Could you check a few things on this model? Use its own coordinates, in mm. Face numbers are marked on the shaded views. Round coordinates to 2 decimals unless told otherwise and drop trailing zeros. Write each loop counter-clockwise with the first axis right and the second up, starting at its lowest first coordinate (ties: lowest second). Pieces come first, ordered by that corner, then holes. Notation, with made-up numbers: (19.25, 57.5) - (75.25, 57.5) arc R31 ccw to (75.25, 84.5) - close; hole circle Ø4 at (62.5, 75). An arc over 180 degrees is marked (long way). Write each question's results on one line, items separated by ' | '. Start each with the question number.
(1) Imagine slicing it at D-D on z = 1. Write out the boundary of the cut face in (x, y) (3 decimals), then the cut area to 3 significant figures.
(2) Imagine slicing it at C-C on y = -6. Write out the boundary of the cut face in (x, z), then the cut area to 3 significant figures.
(3) Imagine slicing it at B-B on x = 25.4. Write out the boundary of the cut face in (y, z) (1 decimal), then the cut area to 3 significant figures.
(4) For P1, Ø8, axis at x = 25.4, y = -9.525, coming from the +Z side; P2, Ø4, axis at x = -6, y = -9.5, coming from the +Z side, each with a flat end and sliding along its axis, tell me the tip position at first contact or that it passes through.
(5) Imagine slicing it at A-A on x = -25.4. Write out the boundary of the cut face in (y, z) (1 decimal), then the cut area to 3 significant figures.
(6) Thinking about a two-plate mould opening in X: for the marked faces 1 and 2, which applies, +X half, -X half, draft (parallel to the pull), parting line (faces both ways), or undercut?
(7) Please list where these lines run through material, in increasing order: line 1 (Y direction, x = -25.4, z = 1.6) (3 decimals); line 2 (Y direction, x = 2, z = 1.45) (3 decimals); line 3 (X direction, y = 8.5, z = 1.8). Write a range as [from, to].
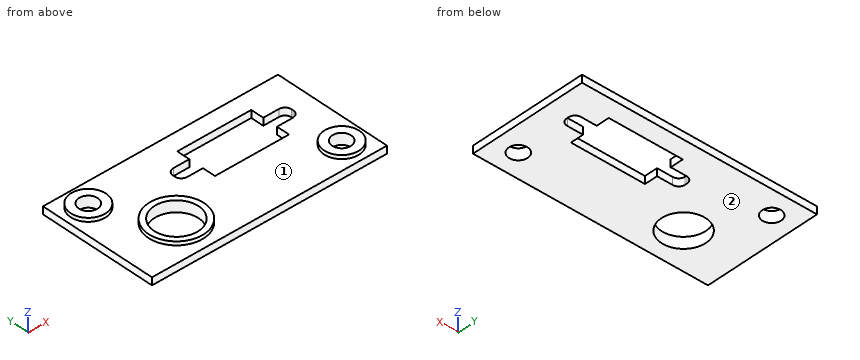
```python
from build123d import *

# Parameters (mm, degrees)
F0_W      = 63.5
F0_H      = 31.75
F1_DEPTH  = 2
F3_R      = 4.7625
F4_DEPTH  = 1
F6_R      = 2.54
F7_DEPTH  = 25.4
F8_W      = 20
F8_H      = 11
F9_DEPTH  = 25
F11_R     = 7.5
F12_DEPTH = 1
F13_R     = 6
F14_DEPTH = 25
F5_R      = 4.7625
F15_DEPTH = 1
F16_R     = 2.54
F17_DEPTH = 25.4
F19_DEPTH = 25


with BuildPart() as f1:
    # F0 (on Top) → F1 (new body)
    with BuildSketch(Plane.XY):
        Rectangle(F0_W, F0_H)
    extrude(amount=F1_DEPTH)

    # F3 (on face) → F4 (join)
    with BuildSketch(Plane.XY.offset(2)):
        with Locations((-25.4, 9.525)):
            Circle(F3_R)
    extrude(amount=F4_DEPTH)

    # F6 (on face) → F7 (cut)
    with BuildSketch(Plane.XY.offset(3)):
        with Locations((-25.4, 9.525)):
            Circle(F6_R)
    extrude(amount=-F7_DEPTH, mode=Mode.SUBTRACT)

    # F8 (on face) → F9 (cut)
    with BuildSketch(Plane.XY.offset(2)):
        with Locations((10, 5.5)):
            Rectangle(F8_W, F8_H)
    extrude(amount=-F9_DEPTH, mode=Mode.SUBTRACT)

    # F11 (on face) → F12 (join)
    with BuildSketch(Plane.XY.offset(2)):
        with Locations((-16, -6)):
            Circle(F11_R)
    extrude(amount=F12_DEPTH)

    # F13 (on face) → F14 (cut)
    with BuildSketch(Plane.XY.offset(3)):
        with Locations((-16, -6)):
            Circle(F13_R)
    extrude(amount=-F14_DEPTH, mode=Mode.SUBTRACT)

    # F5 (on face) → F15 (join)
    with BuildSketch(Plane.XY.offset(2)):
        with Locations((25.4, -9.525)):
            Circle(F5_R)
    extrude(amount=F15_DEPTH)

    # F16 (on face) → F17 (cut)
    with BuildSketch(Plane.XY.offset(3)):
        with Locations((25.4, -9.525)):
            Circle(F16_R)
    extrude(amount=-F17_DEPTH, mode=Mode.SUBTRACT)

    # F18 (on face) → F19 (cut)
    with BuildSketch(Plane.XY.offset(2)):
        with BuildLine():
            Line((6, 3.5), (6, 7.5))
            Line((6, 7.5), (-4.25, 7.5))
            ThreePointArc((-4.25, 7.5), (-5.487437, 6.987437), (-6, 5.75))
            Line((-6, 5.75), (-6, 5.25))
            ThreePointArc((-6, 5.25), (-5.487437, 4.012563), (-4.25, 3.5))
            Line((-4.25, 3.5), (6, 3.5))
        make_face()
        with BuildLine():
            Line((14, 3.5), (24.25, 3.5))
            ThreePointArc((24.25, 3.5), (25.487437, 4.012563), (26, 5.25))
            Line((26, 5.25), (26, 5.75))
            ThreePointArc((26, 5.75), (25.487437, 6.987437), (24.25, 7.5))
            Line((24.25, 7.5), (14, 7.5))
            Line((14, 7.5), (14, 3.5))
        make_face()
    extrude(amount=-F19_DEPTH, mode=Mode.SUBTRACT)


solid = f1.part
```
Response:
1) outline: (-31.75, -15.875) - (31.75, -15.875) - (31.75, 15.875) - (-31.75, 15.875) - close; hole circle Ø5.08 at (-25.4, 9.525); hole circle Ø12 at (-16, -6); hole (-6, 5.25) arc R1.75 ccw to (-4.25, 3.5) - (0, 3.5) - (0, 0) - (20, 0) - (20, 3.5) - (24.25, 3.5) arc R1.75 ccw to (26, 5.25) - (26, 5.75) arc R1.75 ccw to (24.25, 7.5) - (20, 7.5) - (20, 11) - (0, 11) - (0, 7.5) - (-4.25, 7.5) arc R1.75 ccw to (-6, 5.75) - close; hole circle Ø5.08 at (25.4, -9.525) | area: 1,600 mm²
2) outline: (-31.75, 0) - (-22, 0) - (-22, 3) - (-23.5, 3) - (-23.5, 2) - (-31.75, 2) - close; (-10, 0) - (31.75, 0) - (31.75, 2) - (28.6, 2) - (28.6, 3) - (22.2, 3) - (22.2, 2) - (-8.5, 2) - (-8.5, 3) - (-10, 3) - close | area: 112 mm²
3) outline: (-15.9, 0) - (-12.1, 0) - (-12.1, 3) - (-14.3, 3) - (-14.3, 2) - (-15.9, 2) - close; (-7, 0) - (3.9, 0) - (3.9, 2) - (-4.8, 2) - (-4.8, 3) - (-7, 3) - close; (7.1, 0) - (15.9, 0) - (15.9, 2) - (7.1, 2) - close | area: 51.5 mm²
4) P1: z = 3 | P2: z = 2
5) outline: (-15.9, 0) - (7, 0) - (7, 3) - (4.8, 3) - (4.8, 2) - (-15.9, 2) - close; (12.1, 0) - (15.9, 0) - (15.9, 2) - (14.3, 2) - (14.3, 3) - (12.1, 3) - close | area: 57.8 mm²
6) face 1: undercut | face 2: draft
7) line 1: [-15.875, 6.985], [12.065, 15.875] | line 2: [-15.875, 0], [11, 15.875] | line 3: [-31.75, -27.72], [-23.08, 0], [20, 31.75]
